```python
from build123d import *

# Parameters (mm, degrees)
SKETCH1_R               = 12.5
BOSS_EXTRUDE1_DEPTH     = 10
SHELL1_T                = -1
CUT_EXTRUDE1_DEPTH      = 21.310096012
CUT_EXTRUDE1_DEPTH_BACK = 21.310096012
SKETCH2_W               = 15
SKETCH2_H               = 9
SKETCH3_R               = 1
CUT_EXTRUDE2_DEPTH      = 10
SKETCH4_R               = 4
CUT_EXTRUDE3_DEPTH      = 10


with BuildPart() as part:
    # Sketch1 → Boss-Extrude1 (new body)
    with BuildSketch(Plane(origin=(0, 0, 0), x_dir=(1, 0, 0), z_dir=(0, 1, 0))):
        with Locations(Location((0, 0, 0), (0, 0, 270))):
            Circle(SKETCH1_R)
    extrude(amount=BOSS_EXTRUDE1_DEPTH)

    # Shell1
    shell1_openings = [part.faces().sort_by_distance(p)[0] for p in [
        (0, 0, 0),
    ]]
    offset(amount=SHELL1_T, openings=shell1_openings, kind=Kind.INTERSECTION)

    # Sketch2 → Cut-Extrude1 (cut, two sides: drawn at the far end of the back side and taken through both)
    with BuildSketch(Plane.XY.offset(-CUT_EXTRUDE1_DEPTH_BACK)):
        with Locations((0, 4.5)):
            Rectangle(SKETCH2_W, SKETCH2_H)
    extrude(amount=CUT_EXTRUDE1_DEPTH + CUT_EXTRUDE1_DEPTH_BACK, mode=Mode.SUBTRACT)

    # Sketch3 → Cut-Extrude2 (cut)
    with BuildSketch(Plane(origin=(0, 10, 0), x_dir=(1, 0, 0), z_dir=(0, 1, 0))):
        with Locations(Location((-10, 0, 0), (0, 0, 270))):
            Circle(SKETCH3_R)
        with Locations(Location((-6, 0, 0), (0, 0, 270))):
            Circle(SKETCH3_R)
        with Locations(Location((-5, 8.660254038, 0), (0, 0, 270))):
            Circle(SKETCH3_R)
        with Locations(Location((-3, 5.196152423, 0), (0, 0, 270))):
            Circle(SKETCH3_R)
        with Locations(Location((5, 8.660254038, 0), (0, 0, 270))):
            Circle(SKETCH3_R)
        with Locations(Location((3, 5.196152423, 0), (0, 0, 270))):
            Circle(SKETCH3_R)
        with Locations(Location((10, 0, 0), (0, 0, 270))):
            Circle(SKETCH3_R)
        with Locations(Location((6, 0, 0), (0, 0, 270))):
            Circle(SKETCH3_R)
        with Locations(Location((5, -8.660254038, 0), (0, 0, 270))):
            Circle(SKETCH3_R)
        with Locations(Location((3, -5.196152423, 0), (0, 0, 270))):
            Circle(SKETCH3_R)
        with Locations(Location((-5, -8.660254038, 0), (0, 0, 270))):
            Circle(SKETCH3_R)
        with Locations(Location((-3, -5.196152423, 0), (0, 0, 270))):
            Circle(SKETCH3_R)
    extrude(amount=-CUT_EXTRUDE2_DEPTH, mode=Mode.SUBTRACT)

    # Sketch4 → Cut-Extrude3 (cut)
    with BuildSketch(Plane(origin=(0, 10, 0), x_dir=(1, 0, 0), z_dir=(0, 1, 0))):
        with Locations(Location((0, 0, 0), (0, 0, 270))):
            Circle(SKETCH4_R)
    extrude(amount=-CUT_EXTRUDE3_DEPTH, mode=Mode.SUBTRACT)


solid = part.part
```
Verification items for the finished model (mm, model axes). A direction names the side the tool comes from. Coordinates: 2 decimals unless noted, no trailing zeros. Loops run counter-clockwise (first coordinate to the right, second up) from the corner with the lowest first, then second, coordinate; pieces in that order, holes last. Notation, with made-up numbers: (-2, -25) -> (3, -25) arc R18 cw to (3, -11) -> close; hole circle Ø2 at (-25.75, 3.25). An arc over 180 degrees is marked (long way). Put each result on its own line as item: value.
1. Tool access check on faces 1 (the face through (-11.5, 4.4, -0.1)), 2 (the face through (-12, 0, 0)), 3 (the face through (7.5, 4, 9)). Record the directions out of +Z, -Z, +X, -X, +Y, -Y that give a thin tool (end or side, any length) a straight path to the whole face; none if there is none.
Result set:
face 1: -Y
face 2: +Z, -Z, +X, -X, -Y
face 3: +Z, -Z, -Y
2. Thickness scan on line 1 (X direction, y = 9.35, z = 0); line 2 (X direction, y = 4.5, z = 0); line 3 (Z direction, x = 10, y = 1.25). Record the ranges inside material, lowest first.
Result set:
line 1: x = -12.5 to -11, -9 to -7, -5 to -4, 4 to 5, 7 to 9, 11 to 12.5
line 2: x = -12.5 to -11.5, 11.5 to 12.5
line 3: z = -7.5 to -5.68, 5.68 to 7.5
3. Mould release check, pull along X, two halves, no side actions. Record for faces 4 (the face through (-3, 9, -3)), 5 (the face through (12, 0, 0)), 6 (the face through (8.45, 4.93, -9.21)): pulls with the +X half, pulls with the -X half, needs draft (parallel to the pull), parting line crosses it, or undercut.
Result set:
face 4: undercut
face 5: needs draft
face 6: parting line crosses it
4. Section check B-B, the plane x = 0. Record the boundary of the cut face in (y, z).
Result set:
outline: (9, -12.5) -> (10, -12.5) -> (10, -4) -> (9, -4) -> close; (9, 4) -> (10, 4) -> (10, 12.5) -> (9, 12.5) -> close
5. Section check D-D, the plane x = -10. Record the boundary of the cut face in (y, z).
Result set:
outline: (0, -7.5) -> (10, -7.5) -> (10, -1) -> (9, -1) -> (9, -5.68) -> (0, -5.68) -> close; (0, 5.68) -> (9, 5.68) -> (9, 1) -> (10, 1) -> (10, 7.5) -> (0, 7.5) -> close
6. Section check A-A, the plane y = 1.25. Record the boundary of the cut face in (x, z), then the cut area to 3 significant figures.
Result set:
outline: (-7.5, -10) -> (-7.5, -8.72) arc R11.5 cw to (-7.5, 8.72) -> (-7.5, 10) arc R12.5 ccw to start; (7.5, -10) arc R12.5 ccw to (7.5, 10) -> (7.5, 8.72) arc R11.5 cw to (7.5, -8.72) -> close
area: 43.0 mm^2
7. Gauge pin test, flat ends, axial feed: P1, Ø3, axis at x = 3, z = 5.2, coming from the -Y side; P2, Ø1.5, axis at y = 7.5, z = 8, coming from the -X side; P3, Ø1, axis at y = 6, z = 9, coming from the -X side. Record the tip position at first contact, or that the pin passes through.
Result set:
P1: stops at y = 9
P2: stops at x = -10.18
P3: stops at x = -9.17
8. Section check C-C, the plane z = -2.75. Record the boundary of the cut face in (x, y), then the cut area to 3 significant figures.
Result set:
outline: (-12.19, 0) -> (-11.17, 0) -> (-11.17, 9) -> (-2.9, 9) -> (-2.9, 10) -> (-12.19, 10) -> close; (2.9, 9) -> (11.17, 9) -> (11.17, 0) -> (12.19, 0) -> (12.19, 10) -> (2.9, 10) -> close
area: 37.1 mm^2
